```python
from build123d import *

# Parameters (mm, degrees)
SKETCH1_W           = 80.01
SKETCH1_H           = 102.87
BOSS_EXTRUDE1_DEPTH = 3.175
SKETCH2_W           = 3.175
SKETCH2_H           = 6.35
CUT_EXTRUDE1_DEPTH  = 4.175
SKETCH3_W           = 6.35
SKETCH3_H           = 3.175
CUT_EXTRUDE2_DEPTH  = 4.175
SKETCH4_R           = 2.54
SKETCH4_R_2         = 5
CUT_EXTRUDE3_DEPTH  = 4.175


with BuildPart() as part:
    # Sketch1 → Boss-Extrude1 (new body)
    with BuildSketch(Plane(origin=(0, 0, 0), x_dir=(1, 0, 0), z_dir=(0, 1, 0))):
        Rectangle(SKETCH1_W, SKETCH1_H)
    extrude(amount=BOSS_EXTRUDE1_DEPTH)

    # Sketch2 → Cut-Extrude1 (cut, through all)
    with BuildSketch(Plane(origin=(0, 3.175, 0), x_dir=(1, 0, 0), z_dir=(0, 1, 0))):
        with Locations((-38.4175, -38.1)):
            Rectangle(SKETCH2_W, SKETCH2_H)
        with Locations((-38.4175, -25.4)):
            Rectangle(SKETCH2_W, SKETCH2_H)
        with Locations((-38.4175, -12.7)):
            Rectangle(SKETCH2_W, SKETCH2_H)
        with Locations((-38.4175, 0)):
            Rectangle(SKETCH2_W, SKETCH2_H)
        with Locations((-38.4175, 12.7)):
            Rectangle(SKETCH2_W, SKETCH2_H)
        with Locations((-38.4175, 25.4)):
            Rectangle(SKETCH2_W, SKETCH2_H)
        with Locations((38.4175, 25.4)):
            Rectangle(SKETCH2_W, SKETCH2_H)
        with Locations((38.4175, 12.7)):
            Rectangle(SKETCH2_W, SKETCH2_H)
        with Locations((38.4175, 0)):
            Rectangle(SKETCH2_W, SKETCH2_H)
        with Locations((38.4175, -12.7)):
            Rectangle(SKETCH2_W, SKETCH2_H)
        with Locations((38.4175, -25.4)):
            Rectangle(SKETCH2_W, SKETCH2_H)
        with Locations((38.4175, -38.1)):
            Rectangle(SKETCH2_W, SKETCH2_H)
        with Locations((-38.4175, 38.1)):
            Rectangle(SKETCH2_W, SKETCH2_H)
        with Locations((38.4175, 38.1)):
            Rectangle(SKETCH2_W, SKETCH2_H)
    extrude(amount=-CUT_EXTRUDE1_DEPTH, mode=Mode.SUBTRACT)

    # Sketch3 → Cut-Extrude2 (cut, through all)
    with BuildSketch(Plane(origin=(0, 3.175, 0), x_dir=(1, 0, 0), z_dir=(0, 1, 0))):
        with Locations((25.4, 49.8475)):
            Rectangle(SKETCH3_W, SKETCH3_H)
        with Locations((12.7, 49.8475)):
            Rectangle(SKETCH3_W, SKETCH3_H)
        with Locations((0, 49.8475)):
            Rectangle(SKETCH3_W, SKETCH3_H)
        with Locations((-12.7, 49.8475)):
            Rectangle(SKETCH3_W, SKETCH3_H)
        with Locations((-12.7, -49.8475)):
            Rectangle(SKETCH3_W, SKETCH3_H)
        with Locations((0, -49.8475)):
            Rectangle(SKETCH3_W, SKETCH3_H)
        with Locations((12.7, -49.8475)):
            Rectangle(SKETCH3_W, SKETCH3_H)
        with Locations((25.4, -49.8475)):
            Rectangle(SKETCH3_W, SKETCH3_H)
        with Locations((-25.4, -49.8475)):
            Rectangle(SKETCH3_W, SKETCH3_H)
        with Locations((-25.4, 49.8475)):
            Rectangle(SKETCH3_W, SKETCH3_H)
    extrude(amount=-CUT_EXTRUDE2_DEPTH, mode=Mode.SUBTRACT)

    # Sketch4 → Cut-Extrude3 (cut, through all)
    with BuildSketch(Plane(origin=(0, 3.175, 0), x_dir=(1, 0, 0), z_dir=(0, 1, 0))):
        with Locations((0, 35.56)):
            Circle(SKETCH4_R)
        with Locations((17.78, 35.56)):
            Circle(SKETCH4_R_2)
        with Locations((12.7, -22.86)):
            Circle(SKETCH4_R_2)
        with Locations((-12.7, -22.86)):
            Circle(SKETCH4_R_2)
    extrude(amount=-CUT_EXTRUDE3_DEPTH, mode=Mode.SUBTRACT)


solid = part.part
```
For this review, take the finished solid that the model builds, in its own axes (mm). A direction names the side the tool comes from. Give positions to 0.01 mm unless a question says otherwise; leave off trailing zeros. Loops run counter-clockwise (first coordinate to the right, second up) from the corner with the lowest first, then second, coordinate; pieces in that order, holes last. Notation, with made-up numbers: M 63,21 L 71,21 A21 cw 71,35 Z; hole C -16.75,45 d9. An arc over 180 degrees is marked long. One line per item, written item: value. Start each with the question number.
Q1. Machinability: for faces 1 (the face through (38, 2, -3.175)), 2 (the face through (-36.83, 2, -13)), 3 (the face through (3.175, 2, 50)), 4 (the face through (0, 2, -48.26)), which of the approach directions +Z, -Z, +X, -X, +Y, -Y give a long, thin tool a straight path to every point of the face, cutting with its end or side? Answer none if there is none.
Q2. Draft analysis for pull direction X (two halves, no side actions). For faces 5 (the face through (40.005, 2, -32)), 6 (the face through (38, 2, 15.875)), 7 (the face through (25, 2, 48.26)), state which applies: released by +X, released by -X, zero draft, split by the parting line, or undercut.
Q3. Clearance check with flat-ended pins moving along their axes: pin 1 Ø1 at (x, y) = (-13, 2) entering from +Z; pin 2 Ø1.6 at (y, z) = (1.5, 1) entering from -X; pin 3 Ø1 at (x, y) = (-14, 1.5) entering from -Z. State where each tip first meets the part, or that it passes through.
Q4. Add section D-D (x = -27). Give the boundary of the cut face in (y, z) (3 decimals), and give its area (3 significant figures).
Q5. Add section C-C (y = 0.85). Count the separate pieces of the cut face and the enclosed holes in it, and give its area (3 significant figures).
Q6. For L1, parallel to X at y = 1.2, z = -35.56; L2, parallel to X at y = 2.1, z = 22.86; L3, parallel to Z at x = 17.78, y = 0.9 (3 decimals), list the stretches that pass through material, from the lowest coordinate up.
Q7. Add section B-B (x = 0). Give the boundary of the cut face in (y, z) (3 decimals), and give its area (3 significant figures).
Q8. Add section A-A (x = -12.7). Give the boundary of the cut face in (y, z) (3 decimals).
Reply:
1. face 1: +X, +Y, -Y
1. face 2: -X, +Y, -Y
1. face 3: +Z, +Y, -Y
1. face 4: -Z, +Y, -Y
2. face 5: released by +X
2. face 6: zero draft
2. face 7: undercut
3. pin 1: z = 48.26
3. pin 2: x = -36.83
3. pin 3: z = -48.26
4. outline: M 0,-48.26 L 3.175,-48.26 L 3.175,48.26 L 0,48.26 Z
4. area: 306 mm²
5. separate pieces: 1
5. enclosed holes: 4
5. area: 7,490 mm²
6. L1: -36.83 to -2.54, 2.54 to 12.78, 22.78 to 36.83
6. L2: -36.83 to -17.7, -7.7 to 7.7, 17.7 to 36.83
6. L3: -51.435 to -40.56, -30.56 to 51.435
7. outline: M 0,-48.26 L 3.175,-48.26 L 3.175,-38.1 L 0,-38.1 Z; M 0,-33.02 L 3.175,-33.02 L 3.175,48.26 L 0,48.26 Z
7. area: 290 mm²
8. outline: M 0,-48.26 L 3.175,-48.26 L 3.175,17.86 L 0,17.86 Z; M 0,27.86 L 3.175,27.86 L 3.175,48.26 L 0,48.26 Z
